Geometry: see drawing. Coordinates: mm, zero at the bounding-box minimum. Round coordinates to 2 decimals unless told otherwise and drop trailing zeros. Write each loop counter-clockwise with the first axis right and the second up, starting at its lowest first coordinate (ties: lowest second). Pieces come first, ordered by that corner, then holes. Notation, with made-up numbers: M 76,83 L 127,83 A24 ccw 127,110 Z; hole C 23,46 d3. An arc over 180 degrees is marked long. Use a Markdown table: item, result.
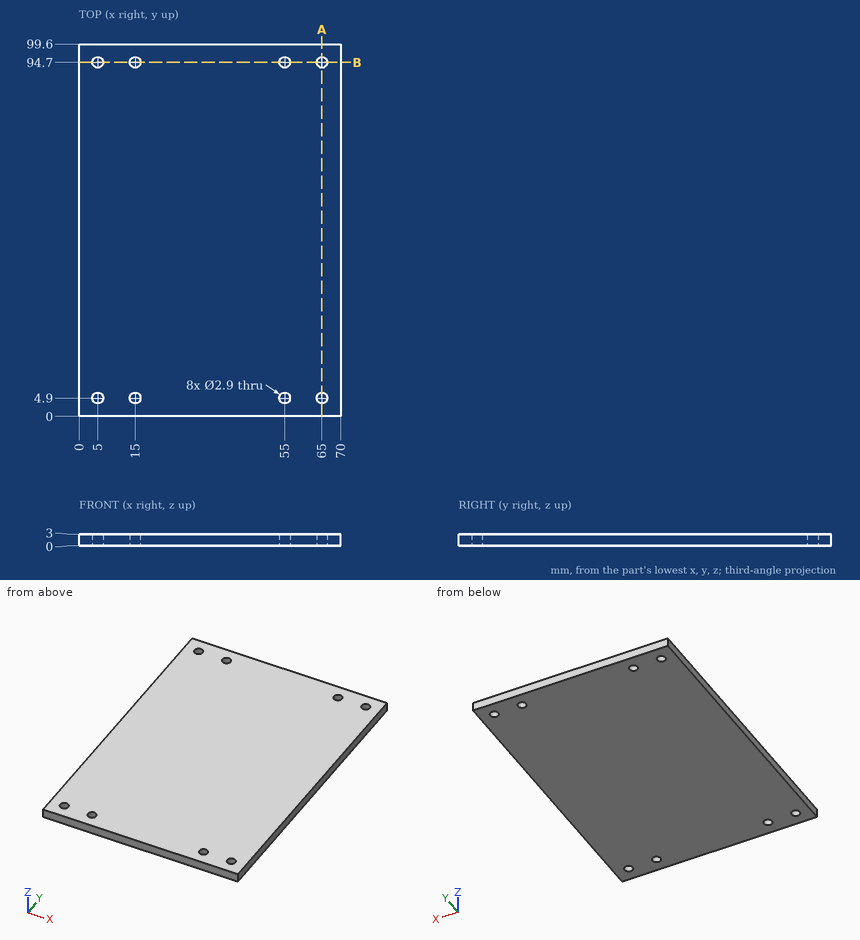
Q1. Section B-B on y = 94.7. Return loops of the section in (x, z).
Results are:
| item | result |
|---|---|
| outline | M 0,0 L 3.55,0 L 3.55,3 L 0,3 Z; M 6.45,0 L 13.55,0 L 13.55,3 L 6.45,3 Z; M 16.45,0 L 53.55,0 L 53.55,3 L 16.45,3 Z; M 56.45,0 L 63.55,0 L 63.55,3 L 56.45,3 Z; M 66.45,0 L 70,0 L 70,3 L 66.45,3 Z |
Q2. Section A-A on x = 65. Return loops of the section in (y, z), plus the area to 3 significant figures.
Results are:
| item | result |
|---|---|
| outline | M 0,0 L 3.45,0 L 3.45,3 L 0,3 Z; M 6.35,0 L 93.25,0 L 93.25,3 L 6.35,3 Z; M 96.15,0 L 99.6,0 L 99.6,3 L 96.15,3 Z |
| area | 281 mm^2 |
Q3. Line query: L1, parallel to X at y = 94.7, z = 1.2; L2, parallel to Y at x = 5, z = 0.8; L3, parallel to Y at x = 54, z = 0.5. Output: solid intervals per line, ascending.
Results are:
| item | result |
|---|---|
| L1 | 0 to 3.55, 6.45 to 13.55, 16.45 to 53.55, 56.45 to 63.55, 66.45 to 70 |
| L2 | 0 to 3.45, 6.35 to 93.25, 96.15 to 99.6 |
| L3 | 0 to 3.85, 5.95 to 93.65, 95.75 to 99.6 |
Q4. First-contact query: pin 1 Ø2.5 at (x, y) = (55, 4.9) entering from -Z. Flat tip, straight axial feed; report the tip coordinate or a pass-through.
Results are:
| item | result |
|---|---|
| pin 1 | through |
